```python
from build123d import *

# Parameters (mm, degrees)
SKICA1_W                = 46
SKICA1_H                = 170.5
SKICA1_R                = 1.5
P_IDAT_VYSUNUT_M1_DEPTH = 3
SKICA2_W                = 36
SKICA2_H                = 160.5
SKICA2_W_2              = 34
SKICA2_H_2              = 158.5
P_IDAT_VYSUNUT_M2_DEPTH = 6


with BuildPart() as part:
    # Skica1 → Přidat vysunutím1 (new body)
    with BuildSketch(Plane.XY):
        with Locations((-17, 72.25)):
            Rectangle(SKICA1_W, SKICA1_H)
        with Locations((-37.5, -10.5)):
            Circle(SKICA1_R, mode=Mode.SUBTRACT)
        with Locations((3.5, -10.5)):
            Circle(SKICA1_R, mode=Mode.SUBTRACT)
        with Locations((3.5, 30.5)):
            Circle(SKICA1_R, mode=Mode.SUBTRACT)
        with Locations((3.5, 71.5)):
            Circle(SKICA1_R, mode=Mode.SUBTRACT)
        with Locations((3.5, 112.5)):
            Circle(SKICA1_R, mode=Mode.SUBTRACT)
        with Locations((3.5, 153.5)):
            Circle(SKICA1_R, mode=Mode.SUBTRACT)
        with Locations((-37.5, 30.5)):
            Circle(SKICA1_R, mode=Mode.SUBTRACT)
        with Locations((-37.5, 71.5)):
            Circle(SKICA1_R, mode=Mode.SUBTRACT)
        with Locations((-37.5, 112.5)):
            Circle(SKICA1_R, mode=Mode.SUBTRACT)
        with Locations((-37.5, 153.5)):
            Circle(SKICA1_R, mode=Mode.SUBTRACT)
    extrude(amount=P_IDAT_VYSUNUT_M1_DEPTH)

    # Skica2 → Přidat vysunutím2 (add)
    with BuildSketch(Plane.XY.offset(3)):
        with Locations((-17, 72.25)):
            Rectangle(SKICA2_W, SKICA2_H)
        with Locations((-17, 72.25)):
            Rectangle(SKICA2_W_2, SKICA2_H_2, mode=Mode.SUBTRACT)
    extrude(amount=-P_IDAT_VYSUNUT_M2_DEPTH)


solid = part.part
```
Model file for the job. Use its own axes, mm. A direction names the side the tool comes from. Coordinates: 2 decimals unless noted, no trailing zeros. Order: outer loops, then holes, each group sorted by start corner. A loop starts at its lowest first (then second) coordinate and runs counter-clockwise, first axis right, second up. Notation, with made-up numbers: (63.5, -4.5) - (83.5, -4.5) arc R18 cw to (83.5, 21.5) - close; hole circle Ø10 at (80.25, 63.25). An arc over 180 degrees is marked (long way). Return JSON: item names as keys, results as strings. Group by question number.
1) Mould opens along Y. For faces 1 (the flat face through (-17, -8, -1)), 2 (the flat face through (6, 71, 1)), 3 (the flat face through (-17, 151.5, -1)) say: released by +Y, released by -Y, zero draft, split by the parting line, or undercut.
2) Tool access for faces 4 (the cylindrical face through (3.305, 154.987, 1.479)), 5 (the flat face through (-17, 152.5, -1)), 6 (the flat face through (-34, 71, -1)), 7 (the flat face through (1, 71, -1)), 8 (the flat face through (-35, 71, -1)): list every direction of +Z, -Z, +X, -X, +Y, -Y with a clear straight run to the whole face (end or side of a thin tool).
3) Saw through at A-A, the plane x = 3.5. Write the cut outline in (y, z), plus the area to 4 significant figures.
4) Saw through at B-B, the plane y = 71.5. Write the cut outline in (x, z).
5) Saw through at C-C, the plane z = -1.2. Write the cut outline in (x, y).
6) Probe line 1 (Y direction, x = -37.5, z = 2.3); line 2 (X direction, y = 71.5, z = 1.2); line 3 (X direction, y = 13, z = -2.3). List the from-to ranges inside material, lowest first. Write a range as from..to.
7) Saw through at D-D, the plane x = -29. Write the cut outline in (y, z), plus the area to 4 significant figures.
8) Flat gauge pins, fed straight in: P1, Ø1.8, axis at x = 3.5, y = 112.5, coming from the +Z side; P2, Ø2.5, axis at x = -18, z = -2, coming from the +Y side; P3, Ø1.5, axis at y = 60, z = -1.5, coming from the -X side; P4, Ø3.5, axis at x = -17.5, z = -2, coming from the -Y side. Where does each tip first touch, or does it go through?
Values found:
{
 "1": {"face 1": "released by -Y", "face 2": "zero draft", "face 3": "undercut"},
 "2": {"face 4": "+Z, -Z", "face 5": "-Z, +X, -X, +Y", "face 6": "-Z", "face 7": "-Z, +X, +Y, -Y", "face 8": "-Z, -X, +Y, -Y"},
 "3": {"outline": "(-13, 0) - (-12, 0) - (-12, 3) - (-13, 3) - close; (-9, 0) - (29, 0) - (29, 3) - (-9, 3) - close; (32, 0) - (70, 0) - (70, 3) - (32, 3) - close; (73, 0) - (111, 0) - (111, 3) - (73, 3) - close; (114, 0) - (152, 0) - (152, 3) - (114, 3) - close; (155, 0) - (157.5, 0) - (157.5, 3) - (155, 3) - close", "area": "466.5 mm²"},
 "4": {"outline": "(-40, 0) - (-39, 0) - (-39, 3) - (-40, 3) - close; (-36, 0) - (-35, 0) - (-35, -3) - (-34, -3) - (-34, 0) - (0, 0) - (0, -3) - (1, -3) - (1, 0) - (2, 0) - (2, 3) - (-36, 3) - close; (5, 0) - (6, 0) - (6, 3) - (5, 3) - close"},
 "5": {"outline": "(-35, -8) - (1, -8) - (1, 152.5) - (-35, 152.5) - close; hole (-34, -7) - (0, -7) - (0, 151.5) - (-34, 151.5) - close"},
 "6": {"line 1": "y = -13..-12, -9..29, 32..70, 73..111, 114..152, 155..157.5", "line 2": "x = -40..-39, -36..2, 5..6", "line 3": "x = -35..-34, 0..1"},
 "7": {"outline": "(-13, 0) - (-8, 0) - (-8, -3) - (-7, -3) - (-7, 0) - (151.5, 0) - (151.5, -3) - (152.5, -3) - (152.5, 0) - (157.5, 0) - (157.5, 3) - (-13, 3) - close", "area": "517.5 mm²"},
 "8": {"P1": "passes through", "P2": "stops at y = 152.5", "P3": "stops at x = -35", "P4": "stops at y = -8"}
}
